Model file for the job. Use its own axes, mm. A direction names the side the tool comes from. Give positions to 0.01 mm unless a question says otherwise; leave off trailing zeros. Loops run counter-clockwise (first coordinate to the right, second up) from the corner with the lowest first, then second, coordinate; pieces in that order, holes last. Notation, with made-up numbers: M 19,49 L 53,49 A25 cw 53,79 Z; hole C 19,-33.5 d9. An arc over 180 degrees is marked long. Answer in a Markdown table with one row per item.
```python
from build123d import *

# Parameters (mm, degrees)
CROQUIS1_W              = 70
CROQUIS1_H              = 105
SALIENTE_EXTRUIR1_DEPTH = 3.175
CROQUIS2_R              = 16.5
SALIENTE_EXTRUIR2_DEPTH = 3.175
CROQUIS3_W              = 26
CROQUIS3_H              = 6
CORTAR_EXTRUIR1_DEPTH   = 3.175
CROQUIS4_W              = 3
CROQUIS4_H              = 11
CORTAR_EXTRUIR2_DEPTH   = 1
CROQUIS5_W              = 66
CROQUIS5_H              = 101
SALIENTE_EXTRUIR3_DEPTH = 25


with BuildPart() as part:
    # Croquis1 → Saliente-Extruir1 (new body)
    with BuildSketch(Plane.XY):
        with Locations((35, -52.5)):
            Rectangle(CROQUIS1_W, CROQUIS1_H)
    extrude(amount=SALIENTE_EXTRUIR1_DEPTH)

    # Croquis2 → Saliente-Extruir2 (add)
    with BuildSketch(Plane.XY.offset(3.175)):
        with Locations((35, -26.25)):
            Circle(CROQUIS2_R)
        with Locations((35, -78.75)):
            Circle(CROQUIS2_R)
    extrude(amount=SALIENTE_EXTRUIR2_DEPTH)

    # Croquis3 → Cortar-Extruir1 (cut)
    with BuildSketch(Plane.XY.offset(6.35)):
        with Locations((35, -9.75)):
            Rectangle(CROQUIS3_W, CROQUIS3_H)
        with Locations((35, -42.75)):
            Rectangle(CROQUIS3_W, CROQUIS3_H)
        with Locations((35, -62.25)):
            Rectangle(CROQUIS3_W, CROQUIS3_H)
        with Locations((35, -95.25)):
            Rectangle(CROQUIS3_W, CROQUIS3_H)
    extrude(amount=-CORTAR_EXTRUIR1_DEPTH, mode=Mode.SUBTRACT)

    # Croquis4 → Cortar-Extruir2 (cut)
    with BuildSketch(Plane.XY.offset(6.35)):
        with Locations((27.5, -29.25)):
            Rectangle(CROQUIS4_W, CROQUIS4_H)
        with Locations((42.5, -29.25)):
            Rectangle(CROQUIS4_W, CROQUIS4_H)
        with BuildLine():
            Line((34.632057675, -19.532945654), (35.367942325, -19.532945654))
            ThreePointArc((35.367942325, -19.532945654), (36.923577244, -18.888580572), (37.567942325, -17.332945654))
            Line((37.567942325, -17.332945654), (37.567942325, -14.967054346))
            Line((37.567942325, -14.967054346), (32.432057675, -14.967054346))
            Line((32.432057675, -14.967054346), (32.432057675, -17.332945654))
            ThreePointArc((32.432057675, -17.332945654), (33.076422756, -18.888580572), (34.632057675, -19.532945654))
        make_face()
        with Locations((42.5, -81.75)):
            Rectangle(CROQUIS4_W, CROQUIS4_H)
        with Locations((27.5, -81.75)):
            Rectangle(CROQUIS4_W, CROQUIS4_H)
        with BuildLine():
            Line((34.632057675, -71.973579429), (35.367942325, -71.973579429))
            ThreePointArc((35.367942325, -71.973579429), (36.923577244, -71.329214348), (37.567942325, -69.773579429))
            Line((37.567942325, -69.773579429), (37.567942325, -67.526420571))
            Line((37.567942325, -67.526420571), (32.432057675, -67.526420571))
            Line((32.432057675, -67.526420571), (32.432057675, -69.773579429))
            ThreePointArc((32.432057675, -69.773579429), (33.076422756, -71.329214348), (34.632057675, -71.973579429))
        make_face()
    extrude(amount=-CORTAR_EXTRUIR2_DEPTH, mode=Mode.SUBTRACT)

    # Croquis5 → Saliente-Extruir3 (add)
    with BuildSketch(Plane(origin=(0, 0, 0), x_dir=(-1, 0, 0), z_dir=(0, 0, -1))):
        with Locations((-35, -52.5)):
            Rectangle(CROQUIS5_W, CROQUIS5_H)
    extrude(amount=SALIENTE_EXTRUIR3_DEPTH)


solid = part.part
```
(1) Saw through at A-A, the plane y = -88.5. Give the cut face in (x, z) (3 decimals).
Established:
| item | result |
|---|---|
| outline | M 0,0 L 2,0 L 2,-25 L 68,-25 L 68,0 L 70,0 L 70,3.175 L 48.311,3.175 L 48.311,6.35 L 21.689,6.35 L 21.689,3.175 L 0,3.175 Z |
(2) Saw through at C-C, the plane z = -1.5. Give the cut face in (x, y), and give its area (3 significant figures).
Established:
| item | result |
|---|---|
| outline | M 2,-103 L 68,-103 L 68,-2 L 2,-2 Z |
| area | 6,670 mm2 |
(3) Which spindle directions (+Z, -Z, +X, -X, +Y, -Y) get a long thin tool onto all of the face, cutting with end or side? Do faces 1 (the flat face through (35, -103, -12)), 2 (the cylindrical face through (51.5, -26.5, 4.7)), 3 (the flat face through (42, -29, 5.35)), 4 (the flat face through (35, -65.25, 5)), 5 (the cylindrical face through (18.5, -78.5, 4.7)). Say none if no direction does.
Established:
| item | result |
|---|---|
| face 1 | -Z, +X, -X, -Y |
| face 2 | +Z, +X |
| face 3 | +Z |
| face 4 | +Z, +X, -X |
| face 5 | +Z, -X |
(4) Saw through at D-D, the plane y = -51. Give the cut face in (x, z) (3 decimals), and give its area (3 significant figures).
Established:
| item | result |
|---|---|
| outline | M 0,0 L 2,0 L 2,-25 L 68,-25 L 68,0 L 70,0 L 70,3.175 L 0,3.175 Z |
| area | 1,870 mm2 |
(5) Mould opens along Y. For faces 6 (the flat face through (68, -53, -12)), 7 (the cylindrical face through (33.06, -18.87, 5.86)), 8 (the flat face through (35, -2, -12)) say: pulls with the +Y half, pulls with the -Y half, needs draft (parallel to the pull), parting line crosses it, or undercut.
Established:
| item | result |
|---|---|
| face 6 | needs draft |
| face 7 | undercut |
| face 8 | pulls with the +Y half |
(6) Flat gauge pins, fed straight in: P1, Ø1.1, axis at y = -27, z = 6, coming from the -X side; P2, Ø2, axis at x = 56.5, z = -20, coming from the +Y side; P3, Ø1.3, axis at x = 34, y = -69.5, coming from the +Z side; P4, Ø3.5, axis at x = 42.5, y = -28.5, coming from the +Z side. Where does each tip first touch, or does it go through?
Established:
| item | result |
|---|---|
| P1 | stops at x = 18.5 |
| P2 | stops at y = -2 |
| P3 | stops at z = 5.35 |
| P4 | stops at z = 6.35 |
(7) Wall check: L1, parallel to Y at x = 32.5, z = 5; L2, parallel to X at y = -80, z = -14.5; L3, parallel to Z at x = 44, y = -58 (3 decimals). Give the ranges that are in metal, low to high.
Established:
| item | result |
|---|---|
| L1 | y = -92.25 to -65.25, -39.75 to -12.75 |
| L2 | x = 2 to 68 |
| L3 | z = -25 to 3.175 |
(8) Saw through at B-B, the plane x = 46. Give the cut face in (y, z) (3 decimals), and give its area (3 significant figures).
Established:
| item | result |
|---|---|
| outline | M -105,0 L -103,0 L -103,-25 L -2,-25 L -2,0 L 0,0 L 0,3.175 L -13.952,3.175 L -13.952,6.35 L -38.548,6.35 L -38.548,3.175 L -66.452,3.175 L -66.452,6.35 L -91.048,6.35 L -91.048,3.175 L -105,3.175 Z |
| area | 3,010 mm2 |
